The model under review builds one solid part; all positions refer to its coordinate system, in mm. A direction names the side the tool comes from. Coordinates: 2 decimals unless noted, no trailing zeros. Loops run counter-clockwise (first coordinate to the right, second up) from the corner with the lowest first, then second, coordinate; pieces in that order, holes last. Notation, with made-up numbers: M -36,-30 L -28,-30 A16 cw -28,-10 Z; hole C 10,67.25 d8. An arc over 180 degrees is marked long. Use one line per item in the form item = value.
```python
from build123d import *

# Parameters (mm, degrees)
SKIZZE2_R                         = 2
AUFSATZ_LINEAR_AUSTRAGEN1_DEPTH   = 6
AUFSATZ_LINEAR_AUSTRAGEN1_2_DEPTH = 6
SKIZZE3_W                         = 22.523994606
SKIZZE3_H                         = 4.003536954
SKIZZE3_W_2                       = 3.011174253
SKIZZE3_H_2                       = 10.396463046
AUFSATZ_LINEAR_AUSTRAGEN2_DEPTH   = 1
SKIZZE4_R                         = 5
AUFSATZ_LINEAR_AUSTRAGEN3_DEPTH   = 1
AUFSATZ_LINEAR_START              = 2
SKIZZE5_R                         = 5
AUFSATZ_LINEAR_AUSTRAGEN4_DEPTH   = 2
SKIZZE6_W                         = 13
SKIZZE6_H                         = 8.996463046
SCHNITT_LINEAR_AUSTRAGEN1_DEPTH   = 4.8
SKIZZE7_W                         = 2.020513934
SKIZZE7_H                         = 22.861740996
SCHNITT_LINEAR_AUSTRAGEN2_DEPTH   = 4.8
SKIZZE8_W                         = 3.011174253
SKIZZE8_H                         = 7.714308529
AUFSATZ_LINEAR_AUSTRAGEN5_DEPTH   = 2


with BuildPart() as part:
    # Skizze2 → Aufsatz-Linear austragen1 (new body)
    with BuildSketch(Plane.XY):
        with Locations((50.173867598, 14.290447118)):
            Circle(SKIZZE2_R)
    extrude(amount=AUFSATZ_LINEAR_AUSTRAGEN1_DEPTH)

    # Skizze3 → Aufsatz-Linear austragen2 (add)
    with BuildSketch(Plane(origin=(0, 0, 0), x_dir=(-1, 0, 0), z_dir=(0, 0, -1))):
        with Locations((-38.911870295, 14.288678641)):
            Rectangle(SKIZZE3_W, SKIZZE3_H)
        with Locations((-29.155460119, 7.088678641)):
            Rectangle(SKIZZE3_W_2, SKIZZE3_H_2)
        with BuildLine():
            Line((-30.661047245, 1.890447118), (-50.173867598, 1.890447118))
            ThreePointArc((-50.173867598, 1.890447118), (-48.759654035, 1.30466068), (-48.173867598, -0.109552882))
            ThreePointArc((-48.173867598, -0.109552882), (-48.759654035, -1.523766445), (-50.173867598, -2.109552882))
            Line((-50.173867598, -2.109552882), (-27.649872992, -2.109552882))
            Line((-27.649872992, -2.109552882), (-27.649872992, 1.890447118))
            Line((-27.649872992, 1.890447118), (-30.661047245, 1.890447118))
        make_face()
    extrude(amount=AUFSATZ_LINEAR_AUSTRAGEN2_DEPTH)



with BuildPart() as body_2:
    # Skizze2 → Aufsatz-Linear austragen1 2 (new body)
    with BuildSketch(Plane.XY):
        with Locations((50.173867598, -0.109552882)):
            Circle(SKIZZE2_R)
    extrude(amount=AUFSATZ_LINEAR_AUSTRAGEN1_2_DEPTH)


with BuildPart() as part_1:
    add(part.part)

    add(body_2.part)  # Aufsatz-Linear austragen3 merges body 2
    # Skizze4 → Aufsatz-Linear austragen3 (add)
    with BuildSketch(Plane(origin=(0, 0, 0), x_dir=(-1, 0, 0), z_dir=(0, 0, -1))):
        with Locations((-50.173867598, -0.109552882)):
            Circle(SKIZZE4_R)
        with Locations((-50.173867598, 14.290447118)):
            Circle(SKIZZE4_R)
    extrude(amount=AUFSATZ_LINEAR_AUSTRAGEN3_DEPTH)

    # Skizze5 → Aufsatz-Linear austragen4 (add)
    with BuildSketch(Plane.XY.offset(AUFSATZ_LINEAR_START)):
        with Locations((50.173867598, 14.290447118)):
            Circle(SKIZZE5_R)
        with Locations((50.173867598, -0.109552882)):
            Circle(SKIZZE5_R)
    extrude(amount=-AUFSATZ_LINEAR_AUSTRAGEN4_DEPTH)

    # Skizze6 → Schnitt-Linear austragen1 (cut)
    with BuildSketch(Plane.XY.offset(2)):
        with Locations((50.161047245, 7.088678641)):
            Rectangle(SKIZZE6_W, SKIZZE6_H)
    extrude(amount=-SCHNITT_LINEAR_AUSTRAGEN1_DEPTH, mode=Mode.SUBTRACT)

    # Skizze7 → Schnitt-Linear austragen2 (cut)
    with BuildSketch(Plane.XY.offset(2)):
        with Locations((55.025561854, 7.141160287)):
            Rectangle(SKIZZE7_W, SKIZZE7_H)
    extrude(amount=-SCHNITT_LINEAR_AUSTRAGEN2_DEPTH, mode=Mode.SUBTRACT)

    # Skizze8 → Aufsatz-Linear austragen5 (add)
    with BuildSketch(Plane.XY):
        with Locations((29.155460119, 7.145531888)):
            Rectangle(SKIZZE8_W, SKIZZE8_H)
    extrude(amount=AUFSATZ_LINEAR_AUSTRAGEN5_DEPTH)


solid = part_1.part
```
1. Add section D-D (y = 14.75). State the section outline as (x, z) points.
Response values:
outline = M 27.65,-1 L 54.02,-1 L 54.02,2 L 52.12,2 L 52.12,6 L 48.23,6 L 48.23,2 L 45.2,2 L 45.2,0 L 27.65,0 Z
2. Add section C-C (x = 29.75). State the section outline as (y, z) points.
Response values:
outline = M -2.11,-1 L 16.29,-1 L 16.29,0 L 11,0 L 11,2 L 3.29,2 L 3.29,0 L -2.11,0 Z
3. Wall thickness on line 1 along Z through (x, y) = (34.5, -0.5); line 2 along X through (y, z) = (8.5, 0.25); line 3 along Y through (x, z) = (52, 3.5): over which ranges is each line inside the solid? List them lowest first. Write a range as from..to.
Response values:
line_1 = -1..0
line_2 = 27.65..30.66
line_3 = -0.93..0.71, 13.47..15.11
4. Add section B-B (z = 1.25). State the section outline as (x, y) points.
Response values:
outline = M 27.65,3.29 L 30.66,3.29 L 30.66,11 L 27.65,11 Z; M 45.97,2.59 A5 ccw 54.02,-3.31 L 54.02,2.59 Z; M 45.97,11.59 L 54.02,11.59 L 54.02,17.49 A5 ccw Z
5. Add section A-A (x = 35.75). State the section outline as (y, z) points, then the cut area to 3 significant figures.
Response values:
outline = M -2.11,-1 L 1.89,-1 L 1.89,0 L -2.11,0 Z; M 12.29,-1 L 16.29,-1 L 16.29,0 L 12.29,0 Z
area = 8.00 mm^2
6. Machinability: for faces 1 (the face through (41, 13, -1)), 2 (the face through (29, 7, 2)), 3 (the face through (36.7, -2.11, -0.5)), 4 (the face through (50, 2.59, 1)), 5 (the face through (52.02, -0.88, 3.97)), which of the approach directions +Z, -Z, +X, -X, +Y, -Y give a long, thin tool a straight path to every point of the face, cutting with its end or side? Answer none if there is none.
Response values:
face_1 = -Z, +X, -X, +Y, -Y
face_2 = +Z, +X, -X, +Y, -Y
face_3 = +Z, -Z, -X, -Y
face_4 = +Z, -Z, +X
face_5 = +Z
7. The part is to be moulded in two halves that separate along Y. For faces 6 (the face through (36.7, 16.29, -0.5)), 7 (the face through (54.015, 0, 1)), 8 (the face through (50, 11.587, 1)), say which applies: pulls with the +Y half, pulls with the -Y half, needs draft (parallel to the pull), parting line crosses it, or undercut.
Response values:
face_6 = pulls with the +Y half
face_7 = needs draft
face_8 = undercut
8. Insertion check: P1, Ø0.5, axis at x = 40.5, z = -0.5, coming from the +Y side; P2, Ø12, axis at x = 51, y = 4.5, coming from the -Z side; P3, Ø0.6, axis at x = 29.5, z = 1.5, coming from the +Y side; P4, Ø1.5, axis at y = 8, z = 0, coming from the +X side. Each pin has a flat end and moves straight along its axis. Give the tip position at first contact, or say it passes through.
Response values:
P1 = 16.29
P2 = -1
P3 = 11
P4 = 30.66
